```python
from build123d import *

# Parameters (mm, degrees)
F0_W     = 127
F0_H     = 88.9
F1_DEPTH = 57.15
F2_R     = 12.7
F3_DEPTH = 57.151
F5_DEPTH = 44.45
F6_R     = 5.08
F7_DEPTH = 25.4


with BuildPart() as f1:
    # F0 (on Front) → F1 (new body)
    with BuildSketch(Plane.XZ):
        with Locations((63.5, 44.45)):
            Rectangle(F0_W, F0_H)
    extrude(amount=F1_DEPTH)

    # F2 (on face) → F3 (cut, through all)
    with BuildSketch(Plane.XZ.offset(57.15)):
        with Locations((63.5, 63.5)):
            Circle(F2_R)
        Polygon((127, 0), (127, 21.59), (76.2, 21.59), (76.2, 12.7), (95.25, 12.7), (95.25, 0), align=None)
        Polygon((50.8, 21.59), (0, 21.59), (0, 0), (31.75, 0), (31.75, 12.7), (50.8, 12.7), align=None)
    extrude(amount=-F3_DEPTH, mode=Mode.SUBTRACT)

    # F4 (on face) → F5 (cut)
    with BuildSketch(Plane.XZ.offset(57.15)):
        with BuildLine():
            Line((15.875, 34.29), (41.828237, 76.74744))
            ThreePointArc((41.828237, 76.74744), (51.076735, 85.654514), (63.5, 88.9))
            Line((63.5, 88.9), (0, 88.9))
            Line((0, 88.9), (0, 34.29))
            Line((0, 34.29), (15.875, 34.29))
        make_face()
        with BuildLine():
            ThreePointArc((63.5, 88.9), (75.923265, 85.654514), (85.171763, 76.74744))
            Line((85.171763, 76.74744), (111.125, 34.29))
            Line((111.125, 34.29), (127, 34.29))
            Line((127, 34.29), (127, 88.9))
            Line((127, 88.9), (63.5, 88.9))
        make_face()
    extrude(amount=-F5_DEPTH, mode=Mode.SUBTRACT)

    # F6 (on face) → F7 (cut)
    with BuildSketch(Plane.XY.offset(88.9)):
        with Locations((63.5, -34.925)):
            Circle(F6_R)
    extrude(amount=-F7_DEPTH, mode=Mode.SUBTRACT)


solid = f1.part
```
The listing builds one solid part. Answer for the finished solid, in the listing's coordinates (mm). A direction names the side the tool comes from. Round coordinates to 2 decimals unless told otherwise and drop trailing zeros. Write each loop counter-clockwise with the first axis right and the second up, starting at its lowest first coordinate (ties: lowest second). Pieces come first, ordered by that corner, then holes. Notation, with made-up numbers: (69, 32.5) -> (103, 32.5) arc R15 ccw to (103, 54.5) -> close; hole circle Ø1 at (-26.75, 10). An arc over 180 degrees is marked (long way). Answer as a JSON object with one key per item and string values. Group by question number.
Q1. Straight lines are drawn through the part: line 1 along Y through (x, z) = (116, 73.5); line 2 along X through (y, z) = (-26, 6.5); line 3 along Z through (x, y) = (115, -43). For each, find the intervals that lie inside material, in ascending order.
Q2. Section B-B (x = 83.5) is taken. Write down the section's boundary in (y, z).
Q3. Section A-A (y = -43) is taken. Write down the section's boundary in (x, z) (3 decimals).
Q4. Which of the six approach directions +Z, -Z, +X, -X, +Y, -Y give full straight-line access (tool end or side, diameter ignored) to faces 1 (the face through (76.2, -29, 17)), 2 (the face through (17, -12.7, 68)), 3 (the face through (119, -35, 34.29)), 4 (the face through (31.75, -29, 6))?
Q5. Section D-D (z = 63.5) is taken. Write down the section's boundary in (x, y), plus the area to 3 significant figures.
Q6. Each of these flat-tipped pins is pushed along its axis until it touches: pin 1 Ø5 at (y, z) = (-7.5, 16) entering from +X; pin 2 Ø4 at (y, z) = (-28.5, 76) entering from -X; pin 3 Ø2 at (y, z) = (-38, 38) entering from +X; pin 4 Ø8 at (x, y) = (39, -27.5) entering from -Z. Where does it stop, or does it pass through?
Q7. Determine the mould class of faces 5 (the face through (0, -9, 40)), 6 (the face through (26, -29, 21.59)), 7 (the face through (68.345, -33.399, 82.116)) for opening direction X: pulls with the +X half, pulls with the -X half, needs draft (parallel to the pull), parting line crosses it, or undercut.
Q8. Section C-C (z = 79) is taken. Write down the section's boundary in (x, y) (3 decimals).
Check values:
{
 "1": {"line 1": "-12.7 to 0", "line 2": "31.75 to 95.25", "line 3": "21.59 to 34.29"},
 "2": {"outline": "(-57.15, 0) -> (0, 0) -> (0, 12.7) -> (-57.15, 12.7) -> close; (-57.15, 21.59) -> (0, 21.59) -> (0, 88.9) -> (-12.7, 88.9) -> (-12.7, 79.16) -> (-57.15, 79.16) -> close"},
 "3": {"outline": "(0, 21.59) -> (50.8, 21.59) -> (50.8, 12.7) -> (31.75, 12.7) -> (31.75, 0) -> (95.25, 0) -> (95.25, 12.7) -> (76.2, 12.7) -> (76.2, 21.59) -> (127, 21.59) -> (127, 34.29) -> (111.125, 34.29) -> (85.172, 76.747) arc R25.4 ccw to (63.5, 88.9) arc R25.4 ccw to (41.828, 76.747) -> (15.875, 34.29) -> (0, 34.29) -> close; hole circle Ø25.4 at (63.5, 63.5)"},
 "4": {"face 1": "+X, +Y, -Y", "face 2": "+Z, -X, -Y", "face 3": "+Z, +X, -Y", "face 4": "-Z, -X, +Y, -Y"},
 "5": {"outline": "(0, -12.7) -> (33.73, -12.7) -> (33.73, -57.15) -> (50.8, -57.15) -> (50.8, 0) -> (0, 0) -> close; (76.2, -57.15) -> (93.27, -57.15) -> (93.27, -12.7) -> (127, -12.7) -> (127, 0) -> (76.2, 0) -> close", "area": "2,810 mm^2"},
 "6": {"pin 1": "x = 76.2", "pin 2": "x = 40.15", "pin 3": "x = 109.47", "pin 4": "z = 0"},
 "7": {"face 5": "pulls with the -X half", "face 6": "needs draft", "face 7": "undercut"},
 "8": {"outline": "(0, -12.7) -> (43.378, -12.7) -> (43.378, -57.15) -> (83.622, -57.15) -> (83.622, -12.7) -> (127, -12.7) -> (127, 0) -> (0, 0) -> close; hole circle Ø10.16 at (63.5, -34.925)"}
}
